Verification items for the finished model (mm, model axes). Face numbers are marked on the shaded views. Coordinates: 2 decimals unless noted, no trailing zeros. Write each loop counter-clockwise with the first axis right and the second up, starting at its lowest first coordinate (ties: lowest second). Pieces come first, ordered by that corner, then holes. Notation, with made-up numbers: M 2.5,37 L 53.5,37 A17 ccw 53.5,51 Z; hole C 44,4 d8. An arc over 180 degrees is marked long. One line per item, written item: value.
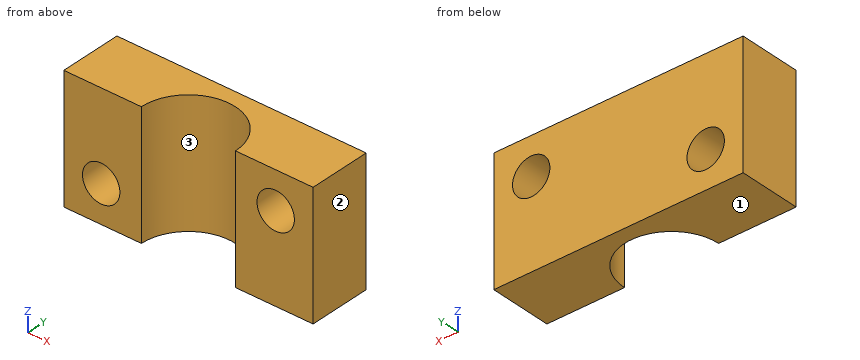
```python
from build123d import *

# Parameters (mm, degrees)
SKETCH1_W           = 20
SKETCH1_H           = 10
BOSS_EXTRUDE1_DEPTH = 5
SKETCH2_R           = 3.775
CUT_EXTRUDE1_DEPTH  = 10
SKETCH3_R           = 1.5
CUT_EXTRUDE2_DEPTH  = 5


with BuildPart() as part:
    # Sketch1 → Boss-Extrude1 (new body)
    with BuildSketch(Plane(origin=(0, 0, 0), x_dir=(1, 0, 0), z_dir=(0, 1, 0))):
        with Locations((-15.016162702, -5.245981532)):
            Rectangle(SKETCH1_W, SKETCH1_H)
    extrude(amount=BOSS_EXTRUDE1_DEPTH)

    # Sketch2 → Cut-Extrude1 (cut)
    with BuildSketch(Plane.XY.offset(10.245981532)):
        with Locations((-15.016162702, 0)):
            Circle(SKETCH2_R)
    extrude(amount=-CUT_EXTRUDE1_DEPTH, mode=Mode.SUBTRACT)

    # Sketch3 → Cut-Extrude2 (cut)
    with BuildSketch(Plane(origin=(0, 5, 0), x_dir=(1, 0, 0), z_dir=(0, 1, 0))):
        with Locations(Location((-22.016162702, -3.245981532, 0), (0, 0, 270))):
            Circle(SKETCH3_R)
        with Locations(Location((-8.016162702, -7.245981532, 0), (0, 0, 270))):
            Circle(SKETCH3_R)
    extrude(amount=-CUT_EXTRUDE2_DEPTH, mode=Mode.SUBTRACT)


solid = part.part
```
Item 1: Scan lines: line 1 (X direction, y = 3.05, z = 6.75); line 2 (X direction, y = 0.5, z = 3.5); line 3 (Z direction, x = -22, y = 1.7). Record each from-to range of solid material in increasing order.
The answers:
line 1: x = -25.02 to -17.24, -12.79 to -9.43, -6.6 to -5.02
line 2: x = -25.02 to -23.49, -20.54 to -18.76, -11.27 to -5.02
line 3: z = 0.25 to 1.75, 4.75 to 10.25
Item 2: Cross-section at A-A, the plane y = 2.05. Enter the section's corners in (x, z), and give its area (3 significant figures).
The answers:
outline: M -25.02,0.25 L -18.19,0.25 L -18.19,10.25 L -25.02,10.25 Z; M -11.85,0.25 L -5.02,0.25 L -5.02,10.25 L -11.85,10.25 Z; hole C -22.02,3.25 d3; hole C -8.02,7.25 d3
area: 122 mm²
Item 3: Draft check along X on the marked faces 1, 2 and 3. Enter one of: released by +X, released by -X, zero draft, split by the parting line, or undercut.
The answers:
face 1: zero draft
face 2: released by +X
face 3: undercut
Item 4: Cross-section at B-B, the plane x = -7.5. Enter the section's corners in (y, z), and give its area (3 significant figures).
The answers:
outline: M 0,0.25 L 5,0.25 L 5,5.84 L 0,5.84 Z; M 0,8.65 L 5,8.65 L 5,10.25 L 0,10.25 Z
area: 35.9 mm²
Item 5: Go/stop test with a flat-tipped pin: P1, Ø1, axis at x = -16, y = 2, coming from the -Z side. Record where the tip stops, or that it passes through.
The answers:
P1: passes through
Item 6: Cross-section at C-C, the plane z = 6.5. Enter the section's corners in (x, y) (3 decimals).
The answers:
outline: M -25.016,0 L -18.791,0 A3.775 cw -11.241,0 L -9.318,0 L -9.318,5 L -25.016,5 Z; M -6.715,0 L -5.016,0 L -5.016,5 L -6.715,5 Z
Item 7: Cross-section at D-D, the plane y = 3.15. Enter the section's corners in (x, z).
The answers:
outline: M -25.02,0.25 L -17.1,0.25 L -17.1,10.25 L -25.02,10.25 Z; M -12.94,0.25 L -5.02,0.25 L -5.02,10.25 L -12.94,10.25 Z; hole C -22.02,3.25 d3; hole C -8.02,7.25 d3
